Source: CAD feature listing. Evaluate the final solid. Frame: model axes, mm. A direction names the side the tool comes from. Round coordinates to 2 decimals unless told otherwise and drop trailing zeros. Loops run counter-clockwise (first coordinate to the right, second up) from the corner with the lowest first, then second, coordinate; pieces in that order, holes last.
(1) Section B-B, the plane z = 3.5. Return the cut outline in (x, y).
(2) Mould query, pull axis Z, two halves, no side actions, for faces 1 (the flat face through (0, 15, 15)), 2 (the cylindrical face through (-5.94, 25.63, -9.32)). Classes: pulls with the +Z half, pulls with the -Z half, needs draft (parallel to the pull), parting line crosses it, or undercut.
(3) Section A-A, the plane x = 0. Return the cut outline in (y, z), plus the area to 3 significant figures.
(4) Material intervals for probe 1 along Y at (x, z) = (16.5, 0) (3 decimals); probe 2 along Z at (x, y) = (0, 48.5), sorted ascending.
(5) Section D-D, the plane x = 13. Return the cut outline in (y, z) (3 decimals), plus the area to 3 significant figures.
(6) First-contact query: pin 1 Ø2 at (x, z) = (9.5, -12.5) entering from -Y; pin 2 Ø1.3 at (x, z) = (-9.19, 9.19) entering from -Y; pin 3 Ø4.5 at (y, z) = (4, 16.5) entering from -X; pin 4 Ø8 at (y, z) = (16, -14.5) entering from -X. Flat tips, straight axial feed; report the tip coordinate or a pass-through.
(7) Set-up query: faces 3 (the cylindrical face through (-0.59, 52.97, 4.46)), 4 (the cylindrical face through (-10.21, 5.07, -9.61)), 5 (the flat face through (0, 0, -13)), 6 (the cylindrical face through (15.94, 30.59, 0.26)), 7 (the flat face through (3, 53.98, 4)). Return all of +Z, -Z, +X, -X, +Y, -Y with unobstructed straight access to the full face (end or side cutting, diameter ignored); none if empty.
(8) Section C-C, the plane y = 17. Return the cut outline in (x, z).
Autodesk Inventor part; units mm, degrees
ref_plane "Work Plane1" through (20, 0, 0) normal (1, 0, 0) x (0, 1, 0)
ref_plane "XZ Plane" through (0, 0, 0) normal (0, 1, 0) x (-1, 0, 0)
ref_plane "XY Plane" through (0, 0, 0) normal (0, 0, 1) x (1, 0, 0)
sketch "Sketch1" plane through (0, 0, 0) normal (0, 1, 0) x (-1, 0, 0)
  circle A0 centre (0, 0) radius 20
  circle A1 centre (0, 0) radius 11.05
  dimension "d0" = 40
  dimension "d1" = 22.1
extrude "Extrusion1" add sketch "Sketch1" along normal blind 51.98
sketch "Sketch2" plane through (0, 0, 0) normal (0, -1, 0) x (1, 0, 0)
  circle A0 centre (0, 0) radius 13
  line L0 (0, 0) -> (9.1924, 0)
  line L1 (9.1924, 0) -> (9.1924, -9.1924)
  line L2 (9.1924, -9.1924) -> (0, -9.1924)
  line L3 (0, -9.1924) -> (0, 0)
  dimension "d4" = 26
  dimension "d5" = 9.1924
hole "Hole1" at (9.1924, 0, -9.1924) direction (0, 1, 0) diameter 2.2 depth 10 tip angle 118
pattern_circular "Circular Pattern1" count 4 over 360 about axis through (0, 0, 0) along (0, 1, 0) of "Hole1"
thread "Thread1"
thread "Thread3"
thread "Thread4"
thread "Thread5"
sketch "Sketch3" plane through (0, 51.98, 0) normal (0, 1, 0) x (1, 0, 0)
  circle A0 centre (0, 0) radius 20
  circle A1 centre (0, 0) radius 4.5
  dimension "d26" = 40
  dimension "d27" = 9
extrude "Extrusion2" add sketch "Sketch3" along normal blind 2
sketch "Sketch4" plane through (0, 53.98, 0) normal (0, 1, 0) x (1, 0, 0)
  point P0 (0, 0)
sketch "Sketch5" plane through (0, 53.98, 0) normal (0, 1, 0) x (1, 0, 0)
  circle A0 centre (0, 0) radius 6.75
  circle A1 centre (0, 0) radius 20
  dimension "d30" = 13.5
  dimension "d31" = 40
extrude "Extrusion3" add sketch "Sketch5" along normal blind 12
thread "Thread6"
sketch "Sketch8" plane through (0, 0, 0) normal (0, -1, 0) x (1, 0, 0)
  point P0 (0, 0)
sketch "Sketch9" plane through (0, 0, 0) normal (0, -1, 0) x (1, 0, 0)
  line L0 (0, 9.7277) -> (2.5, 9.7277)
  line L1 (2.5, 9.7277) -> (2.5, 16.3855)
  line L2 (2.5, 16.3855) -> (0, 16.3855)
  line L3 (0, 16.3855) -> (0, 9.7277)
  line L4 (0, 9.7277) -> (-2.5, 9.7277)
  line L5 (-2.5, 9.7277) -> (-2.5, 16.3855)
  line L6 (-2.5, 16.3855) -> (0, 16.3855)
  line L7 (0, 16.3855) -> (0, 9.7277)
  point P0 (0, 0)
  dimension "d54" = 2.5
  dimension "d55" = 2.5
extrude "Extrusion4" cut sketch "Sketch9" against normal blind 15
sketch "Sketch10" plane through (0, 0, 0) normal (1, 0, 0) x (0, 1, 0)
  point P0 (0, 0)
ref_plane "Work Plane1" through (20, 0, 0) normal (1, 0, 0) x (0, 1, 0)
sketch "Sketch15" plane through (0, 0, 0) normal (0, -1, 0) x (1, 0, 0)
  line L0 (2.5024, 10.6669) -> (-2.5, 10.6669)
  line L1 (-2.5, 10.6669) -> (-2.5, 24.5822)
  line L2 (-2.5, 24.5822) -> (2.5024, 24.5822)
  line L3 (2.5024, 24.5822) -> (2.5024, 10.6669)
  point P0 (0, 0)
extrude "Extrusion5" cut sketch "Sketch15" against normal blind 15
sketch "Sketch18" plane through (20, 0, 0) normal (1, 0, 0) x (0, 1, 0)
  line L0 (0, 0) -> (7.575, 0)
  line L1 (7.575, 0) -> (32.575, 0)
  line L2 (32.575, 0) -> (57.575, 0)
  dimension "d129" = 12.8
  dimension "d102" = 7.575
  dimension "d103" = 25
  dimension "d104" = 25
  dimension "d105" = 180
hole "Hole6" at (20, 57.575, 0) direction (-1, 0, 0) diameter 4 depth 8 tip angle 118
hole "Hole7" at (20, 7.575, 0) at (20, 32.575, 0) direction (-1, 0, 0) diameter 4 depth 8 tip angle 118
thread "Thread7"
thread "Thread8"
thread "Thread9"
sketch "Sketch19" plane through (0, 53.98, 0) normal (0, 1, 0) x (1, 0, 0)
  circle A0 centre (0, 0) radius 6.75
  circle A1 centre (0, 0) radius 6.4
  dimension "d128" = 13.5
  dimension "d129" = 12.8
extrude "Extrusion6" add sketch "Sketch19" along normal blind 2
thread "Thread11"
equation "\"d43\" = 60deg"
equation "\"Sketch6_Pitch\" = 0.5"
properties part number "enclosire17ghz"
Output values:
1. outline: (-19.69, 0) - (-10.48, 0) - (-10.48, 51.98) - (-2.83, 51.98) - (-2.83, 53.98) - (-5.36, 53.98) - (-5.36, 55.98) - (-5.77, 55.98) - (-5.77, 65.98) - (-19.69, 65.98) - close; (2.83, 51.98) - (10.48, 51.98) - (10.48, 0) - (19.69, 0) - (19.69, 65.98) - (5.77, 65.98) - (5.77, 55.98) - (5.36, 55.98) - (5.36, 53.98) - (2.83, 53.98) - close
2. face 1: needs draft
2. face 2: undercut
3. outline: (0, -20) - (65.98, -20) - (65.98, -6.75) - (55.98, -6.75) - (55.98, -6.4) - (53.98, -6.4) - (53.98, -4.5) - (51.98, -4.5) - (51.98, -11.05) - (0, -11.05) - close; (15, 11.05) - (51.98, 11.05) - (51.98, 4.5) - (53.98, 4.5) - (53.98, 6.4) - (55.98, 6.4) - (55.98, 6.75) - (65.98, 6.75) - (65.98, 20) - (15, 20) - close
3. area: 1,180 mm2
4. probe 1: y = 0 to 5.575, 9.575 to 30.575, 34.575 to 55.575, 59.575 to 65.98
4. probe 2: z = -20 to -11.05, 11.05 to 20
5. outline: (0, -15.199) - (65.98, -15.199) - (65.98, 15.199) - (0, 15.199) - close; hole circle Ø4 at (7.575, 0); hole circle Ø4 at (32.575, 0); hole circle Ø4 at (57.575, 0)
5. area: 1,970 mm2
6. pin 1: stops at y = 0
6. pin 2: stops at y = 10.27
6. pin 3: stops at x = -14.03
6. pin 4: stops at x = -17.02
7. face 3: +Y, -Y
7. face 4: -Y
7. face 5: +Z, -Z, +X, -X, -Y
7. face 6: +X
7. face 7: +Y
8. outline: circle Ø40 at (0, 0); hole circle Ø22.1 at (0, 0)
